Geometry check sheet. Reference: the model listing, model coordinates, mm. A direction names the side the tool comes from. Give positions to 0.01 mm unless a question says otherwise; leave off trailing zeros. Order: outer loops, then holes, each group sorted by start corner. A loop starts at its lowest first (then second) coordinate and runs counter-clockwise, first axis right, second up. Notation, with made-up numbers: M -26.5,59.25 L 12.5,59.25 A33 ccw 12.5,87.25 Z; hole C -10.75,9 d6. An arc over 180 degrees is marked long. Put each result on its own line as item: value. Start each with the question number.
Q1. Section check A-A on x = 6. Record the cut outline in (y, z), then the cut area to 3 significant figures.
Q2. Mould release check, pull along X, two halves, no side actions. Record for faces 5 (the flat face through (29.609, 2.218, -29.788)), 6 (the cylindrical face through (-35.037, 2.218, 12.519)), 7 (the flat face through (0, 3.5, -13)): +X half, -X half, draft (parallel to the pull), parting line (faces both ways), or undercut.
Q3. Access from +Z, -Z, +X, -X, +Y, -Y to the whole of each face (thin tool, end or side, straight path). Record for faces 1 (the flat face through (-35.6, 2.2, -18.6)), 2 (the flat face through (-18.71, 2.22, -35.61)), 3 (the flat face through (0, 2, -10)), 4 (the flat face through (35.61, 2.22, -18.71)).
Q4. Material ranges on L1, parallel to Z at x = 3.5, y = 0.55; L2, parallel to Z at x = 7, y = 2; L3, parallel to Z at x = 31, y = 1.6, recorded low to high.
Q5. Section check B-B on z = -3.5. Record the cut outline in (x, y), then the cut area to 4 significant figures.
Q6. Section check C-C on z = 19. Record the cut outline in (x, y).
Q7. Section check D-D on y = 0.9. State how many separate pieces and enclosed holes the cut face has, then the cut area to 3 significant figures.
Q8. Go/stop test with flat-tipped pins: pin 1 (0.9 mm diameter, centred on y = 1, z = -22, fed in from -X); pin 2 (2.5 mm diameter, centred on x = 22.63, z = -31.11, fed in from +Y); pin 3 (1.6 mm diameter, centred on y = 1.5, z = -18.5, fed in from -X); pin 4 (2 mm diameter, centred on y = 2, z = -6, fed in from -X). Record where each tip stops, or that it passes through.
```python
from build123d import *

# Parameters (mm, degrees)
SKETCH2_R           = 1.6
BOSS_EXTRUDE1_DEPTH = 4.5
CUT_EXTRUDE1_DEPTH  = 1
FILLET2_R           = 30
CUT_EXTRUDE4_DEPTH  = 52.119956964
SKETCH11_W          = 35
SKETCH11_H          = 20
CUT_EXTRUDE5_DEPTH  = 52.119956964


with BuildPart() as part:
    # Sketch2 → Boss-Extrude1 (new body)
    with BuildSketch(Plane(origin=(0, 0, 0), x_dir=(1, 0, 0), z_dir=(0, 1, 0))):
        Polygon((-12.5, 35), (12.5, 35), (23.334523779, 36.062445841), (36.062445841, 23.334523779), (35, 12.5), (35, -12.5), (36.062445841, -23.334523779), (23.334523779, -36.062445841), (12.5, -35), (-12.5, -35), (-23.334523779, -36.062445841), (-36.062445841, -23.334523779), (-35, -12.5), (-35, 12.5), (-36.062445841, 23.334523779), (-23.334523779, 36.062445841), align=None)
        with Locations(Location((22.627416998, 31.112698372, 0), (0, 0, 270))):
            Circle(SKETCH2_R, mode=Mode.SUBTRACT)
        with Locations(Location((31.112698372, 22.627416998, 0), (0, 0, 270))):
            Circle(SKETCH2_R, mode=Mode.SUBTRACT)
        with Locations(Location((22.627416998, -31.112698372, 0), (0, 0, 270))):
            Circle(SKETCH2_R, mode=Mode.SUBTRACT)
        with Locations(Location((31.112698372, -22.627416998, 0), (0, 0, 270))):
            Circle(SKETCH2_R, mode=Mode.SUBTRACT)
        with Locations(Location((-31.112698372, -22.627416998, 0), (0, 0, 270))):
            Circle(SKETCH2_R, mode=Mode.SUBTRACT)
        with Locations(Location((-22.627416998, -31.112698372, 0), (0, 0, 270))):
            Circle(SKETCH2_R, mode=Mode.SUBTRACT)
        with Locations(Location((-22.627416998, 31.112698372, 0), (0, 0, 270))):
            Circle(SKETCH2_R, mode=Mode.SUBTRACT)
        with Locations(Location((-31.112698372, 22.627416998, 0), (0, 0, 270))):
            Circle(SKETCH2_R, mode=Mode.SUBTRACT)
    extrude(amount=BOSS_EXTRUDE1_DEPTH)

    # Sketch3 → Cut-Extrude1 (cut)
    with BuildSketch(Plane(origin=(0, 4.5, 0), x_dir=(1, 0, 0), z_dir=(0, 1, 0))):
        Polygon((-17.669047558, 29), (21.911688245, 29), (29, 21.911688245), (29, -17.669047558), (17.669047558, -29), (-17.669047558, -29), (-29, -17.669047558), (-29, 17.669047558), align=None)
    extrude(amount=-CUT_EXTRUDE1_DEPTH, mode=Mode.SUBTRACT)

    # Fillet2
    # the kernel refuses this fillet: 30 mm, written as the material it adds along each edge
    with BuildSketch(Plane(origin=(-12.5, 0, -35), x_dir=(1, 0, 0), z_dir=(0, 1, 0))) as fillet2_piece_1:
        with BuildLine():
            CenterArc((FILLET2_R * 0.0489132680018, FILLET2_R), FILLET2_R, 264.399415997, 5.600584003)
            Line((-FILLET2_R * 0.0486797758844, FILLET2_R * 0.00477359471072), (0, 0))
            Line((0, 0), (FILLET2_R * 0.0489132680018, 0))
        make_face()
    extrude(amount=4.5)
    with BuildSketch(Plane(origin=(12.5, 0, -35), x_dir=(-1, 0, 0), z_dir=(0, 1, 0)), Plane(origin=(35, 0, -12.5), x_dir=(0.09759304388620155, 0, -0.9952264052892819), z_dir=(0, 1, 0)), Plane(origin=(35, 0, 12.5), x_dir=(0, 0, -1), z_dir=(0, 1, 0)), Plane(origin=(12.5, 0, 35), x_dir=(0.9952264052892817, 0, 0.09759304388620309), z_dir=(0, 1, 0)), Plane(origin=(-12.5, 0, 35), x_dir=(1, 0, 0), z_dir=(0, 1, 0)), Plane(origin=(-35, 0, 12.5), x_dir=(-0.09759304388619769, 0, 0.9952264052892822), z_dir=(0, 1, 0)), Plane(origin=(-35, 0, -12.5), x_dir=(0, 0, 1), z_dir=(0, 1, 0))) as fillet2_piece_2:
        with BuildLine():
            CenterArc((FILLET2_R * 0.048913268002, -FILLET2_R), FILLET2_R, 90, 5.600584003)
            Line((-FILLET2_R * 0.0486797758846, -FILLET2_R * 0.00477359471075), (0, 0))
            Line((0, 0), (FILLET2_R * 0.048913268002, 0))
        make_face()
    extrude(amount=4.5)

    # Sketch10 → Cut-Extrude4 (cut, through all)
    with BuildSketch(Plane(origin=(0, 3.5, 0), x_dir=(1, 0, 0), z_dir=(0, 1, 0))):
        with BuildLine():
            Line((-1.5, 20), (-1.5, 18))
            ThreePointArc((-1.5, 18), (-1.646446609, 17.646446609), (-2, 17.5))
            Line((-2, 17.5), (-7, 17.5))
            ThreePointArc((-7, 17.5), (-7.353553391, 17.646446609), (-7.5, 18))
            Line((-7.5, 18), (-7.5, 27))
            ThreePointArc((-7.5, 27), (-7.353553391, 27.353553391), (-7, 27.5))
            Line((-7, 27.5), (7, 27.5))
            ThreePointArc((7, 27.5), (7.353553391, 27.353553391), (7.5, 27))
            Line((7.5, 27), (7.5, 18))
            ThreePointArc((7.5, 18), (7.353553391, 17.646446609), (7, 17.5))
            Line((7, 17.5), (2, 17.5))
            ThreePointArc((2, 17.5), (1.646446609, 17.646446609), (1.5, 18))
            Line((1.5, 18), (1.5, 20))
            ThreePointArc((1.5, 20), (1.646446609, 20.353553391), (2, 20.5))
            Line((2, 20.5), (4.5, 20.5))
            ThreePointArc((4.5, 20.5), (4.853553391, 20.646446609), (5, 21))
            Line((5, 21), (5, 24))
            ThreePointArc((5, 24), (4.853553391, 24.353553391), (4.5, 24.5))
            Line((4.5, 24.5), (-4.5, 24.5))
            ThreePointArc((-4.5, 24.5), (-4.853553391, 24.353553391), (-5, 24))
            Line((-5, 24), (-5, 21))
            ThreePointArc((-5, 21), (-4.853553391, 20.646446609), (-4.5, 20.5))
            Line((-4.5, 20.5), (-2, 20.5))
            ThreePointArc((-2, 20.5), (-1.646446609, 20.353553391), (-1.5, 20))
        make_face()
        with BuildLine():
            Line((-2, -20.5), (-4.5, -20.5))
            ThreePointArc((-4.5, -20.5), (-4.853553391, -20.646446609), (-5, -21))
            Line((-5, -21), (-5, -24))
            ThreePointArc((-5, -24), (-4.853553391, -24.353553391), (-4.5, -24.5))
            Line((-4.5, -24.5), (4.5, -24.5))
            ThreePointArc((4.5, -24.5), (4.853553391, -24.353553391), (5, -24))
            Line((5, -24), (5, -21))
            ThreePointArc((5, -21), (4.853553391, -20.646446609), (4.5, -20.5))
            Line((4.5, -20.5), (2, -20.5))
            ThreePointArc((2, -20.5), (1.646446609, -20.353553391), (1.5, -20))
            Line((1.5, -20), (1.5, -18))
            ThreePointArc((1.5, -18), (1.646446609, -17.646446609), (2, -17.5))
            Line((2, -17.5), (7, -17.5))
            ThreePointArc((7, -17.5), (7.353553391, -17.646446609), (7.5, -18))
            Line((7.5, -18), (7.5, -27))
            ThreePointArc((7.5, -27), (7.353553391, -27.353553391), (7, -27.5))
            Line((7, -27.5), (-7, -27.5))
            ThreePointArc((-7, -27.5), (-7.353553391, -27.353553391), (-7.5, -27))
            Line((-7.5, -27), (-7.5, -18))
            ThreePointArc((-7.5, -18), (-7.353553391, -17.646446609), (-7, -17.5))
            Line((-7, -17.5), (-2, -17.5))
            ThreePointArc((-2, -17.5), (-1.646446609, -17.646446609), (-1.5, -18))
            Line((-1.5, -18), (-1.5, -20))
            ThreePointArc((-1.5, -20), (-1.646446609, -20.353553391), (-2, -20.5))
        make_face()
    extrude(amount=-CUT_EXTRUDE4_DEPTH, mode=Mode.SUBTRACT)

    # Sketch11 → Cut-Extrude5 (cut, through all)
    with BuildSketch(Plane(origin=(0, 3.5, 0), x_dir=(1, 0, 0), z_dir=(0, 1, 0))):
        Rectangle(SKETCH11_W, SKETCH11_H)
    extrude(amount=-CUT_EXTRUDE5_DEPTH, mode=Mode.SUBTRACT)


solid = part.part
```
Results found:
1. outline: M 0,-35 L 4.5,-35 L 4.5,-29 L 3.5,-29 L 3.5,-27.5 L 0,-27.5 Z; M 0,-17.5 L 3.5,-17.5 L 3.5,-10 L 0,-10 Z; M 0,10 L 3.5,10 L 3.5,17.5 L 0,17.5 Z; M 0,27.5 L 3.5,27.5 L 3.5,29 L 4.5,29 L 4.5,35 L 0,35 Z
1. area: 117 mm^2
2. face 5: +X half
2. face 6: -X half
2. face 7: undercut
3. face 1: -X, +Y, -Y
3. face 2: -Z, +Y, -Y
3. face 3: +Y, -Y
3. face 4: +X, +Y, -Y
4. L1: z = -35 to -27.5, -24.5 to -20.5, -17.5 to -10, 10 to 17.5, 20.5 to 24.5, 27.5 to 35
4. L2: z = -35 to -27.5, -17.5 to -10, 10 to 17.5, 27.5 to 35
4. L3: z = -28.4 to -24.22, -21.03 to 21.03, 24.22 to 28.4
5. outline: M -35,0 L -17.5,0 L -17.5,3.5 L -29,3.5 L -29,4.5 L -35,4.5 Z; M 17.5,0 L 35,0 L 35,4.5 L 29,4.5 L 29,3.5 L 17.5,3.5 Z
5. area: 134.5 mm^2
6. outline: M -35.64,0 L -7.5,0 L -7.5,3.5 L -27.67,3.5 L -27.67,4.5 L -35.64,4.5 Z; M -1.5,0 L 1.5,0 L 1.5,3.5 L -1.5,3.5 Z; M 7.5,0 L 35.64,0 L 35.64,4.5 L 27.67,4.5 L 27.67,3.5 L 7.5,3.5 Z
7. separate pieces: 1
7. enclosed holes: 11
7. area: 3,760 mm^2
8. pin 1: stops at x = -35.98
8. pin 2: passes through
8. pin 3: stops at x = -35.67
8. pin 4: stops at x = -35
